from build123d import *

# Parameters (mm, degrees)
F_10_24_TAPPED_HOLE3_D                      = 3.75000012
F_10_24_TAPPED_HOLE4_D                      = 3.75000012
F_10_24_TAPPED_HOLE5_D                      = 4.499991
CBORE_FOR_M5_CHEESE_HEAD_SCREW1_D           = 5.5
CBORE_FOR_M5_CHEESE_HEAD_SCREW1_CBORE_D     = 9.5
CBORE_FOR_M5_CHEESE_HEAD_SCREW1_CBORE_DEPTH = 3.3


with BuildPart() as part:
    # Sketch1 → Revolve1 (revolve)
    with BuildSketch(Plane.XY):
        Polygon((0, 0), (57, 0), (57, -190), (104, -190), (104, -185), (63, -185), (63, 8), (0, 8), align=None)
    revolve(axis=Axis((104, -190, 0), (0, 1, 0)))

    # #10-24 Tapped Hole3 (through all)
    with Locations(Plane(origin=(0, 8, 0), x_dir=(1, 0, 0), z_dir=(0, 1, 0))):
        with Locations((146.346, 30.48), (197.654, 30.48), (197.654, -30.48), (146.346, -30.48)):
            Hole(F_10_24_TAPPED_HOLE3_D / 2)

    # #10-24 Tapped Hole4 (through all)
    with Locations(Plane(origin=(0, 8, 0), x_dir=(1, 0, 0), z_dir=(0, 1, 0))):
        with Locations((28, 0)):
            Hole(F_10_24_TAPPED_HOLE4_D / 2)

    # #10-24 Tapped Hole5 (through all)
    with Locations(Plane(origin=(0, 8, 0), x_dir=(1, 0, 0), z_dir=(0, 1, 0))):
        with Locations((12.5, 15.5), (43.5, 15.5), (43.5, -15.5), (12.5, -15.5)):
            Hole(F_10_24_TAPPED_HOLE5_D / 2)

    # CBORE for M5 Cheese Head Screw1 (through all)
    with Locations(Plane(origin=(0, -190, 0), x_dir=(-1, 0, 0), z_dir=(0, -1, 0))):
        with Locations((-79, -25), (-79, 25), (-129, 25), (-129, -25)):
            CounterBoreHole(CBORE_FOR_M5_CHEESE_HEAD_SCREW1_D / 2, CBORE_FOR_M5_CHEESE_HEAD_SCREW1_CBORE_D / 2, CBORE_FOR_M5_CHEESE_HEAD_SCREW1_CBORE_DEPTH)


solid = part.part
Geometry check sheet. Reference: the model listing, model coordinates, mm. A direction names the side the tool comes from. Give positions to 0.01 mm unless a question says otherwise; leave off trailing zeros. Loops run counter-clockwise (first coordinate to the right, second up) from the corner with the lowest first, then second, coordinate; pieces in that order, holes last. Notation, with made-up numbers: (83.5, 71) -> (128.5, 71) arc R22 ccw to (128.5, 106) -> close; hole circle Ø9 at (-32, -3.5). An arc over 180 degrees is marked (long way). Answer in a Markdown table with one row per item. Add a question column.
1) Gauge pin test, flat ends, axial feed: P1, Ø2.5, axis at x = 12.5, z = -15.5, coming from the +Y side (1 decimal); P2, Ø10, axis at x = 122.5, y = -116.5, coming from the -Z side; P3, Ø4, axis at x = 136, z = -53.5, coming from the -Y side; P4, Ø9, axis at x = 129, z = 25, coming from the +Y side. Record the tip position at first contact, or that the pin passes through.
2) Cross-section at C-C on x = 36. Record the boundary of the cut face in (y, z).
3) Set-up check for faces 1 (the face through (64.893, -87.149, 12.315)), 2 (the face through (124.47, -188.37, -26.43)), 3 (the face through (131.62, -185.84, -25.83)): record each of +Z, -Z, +X, -X, +Y, -Y from which the full face is reachable in a straight line by a thin tool's end or side.
4) Cross-section at A-A on x = 104. Record the boundary of the cut face in (y, z), and give its area (3 significant figures).
5) Material ranges on probe 1 along Z at (x, y) = (129, -185.4); probe 2 along X at (y, z) = (3, -15); probe 3 along X at (y, z) = (3, 30), recorded low to high. Write a range as from..to.
6) Cross-section at B-B on y = -122.5. Record the boundary of the cut face in (x, z).
7) Draft check along Z on faces 4 (the face through (150.955, -96.33, 2.067)), 5 (the face through (105, -190, 1)), 6 (the face through (131.62, -185.84, 24.17)). Enter one of: pulls with the +Z half, pulls with the -Z half, needs draft (parallel to the pull), parting line crosses it, or undercut.
Outcome:
| question | item | result |
|---|---|---|
| 1 | P1 | passes through |
| 1 | P2 | stops at z = -45.02 |
| 1 | P3 | stops at y = 0 |
| 1 | P4 | stops at y = -185 |
| 2 | outline | (0, -78.69) -> (8, -78.69) -> (8, 78.69) -> (0, 78.69) -> close |
| 3 | face 1 | +Y |
| 3 | face 2 | -Y |
| 3 | face 3 | +Y, -Y |
| 4 | outline | (-190, -47) -> (0, -47) -> (0, -104) -> (8, -104) -> (8, -41) -> (-185, -41) -> (-185, 41) -> (8, 41) -> (8, 104) -> (0, 104) -> (0, 47) -> (-190, 47) -> close |
| 4 | area | 3,700 mm^2 |
| 5 | probe 1 | z = -39.8..-27.75, -22.25..22.25, 27.75..39.8 |
| 5 | probe 2 | x = 1.09..10.31, 14.69..41.31, 45.69..65.84, 142.16..206.91 |
| 5 | probe 3 | x = 4.42..76.05, 131.95..144.53, 148.16..195.84, 199.47..203.58 |
| 6 | outline | circle Ø94 at (104, 0); hole circle Ø82 at (104, 0) |
| 7 | face 4 | parting line crosses it |
| 7 | face 5 | needs draft |
| 7 | face 6 | undercut |
